```python
from build123d import *

# Parameters (mm, degrees)
SKETCH_2_W           = 80
SKETCH_2_H           = 34
SKETCH_2_R           = 4.05
EXTRUDE_1_DEPTH      = 8
SKETCH_3_R           = 2.55
CUT_EXTRUDE_1_DEPTH  = 88.292611371
CUT_EXTRUDE_2_DEPTH  = 88.292611371
SKETCH_5_R           = 1.55
CUT_EXTRUDE_3_DEPTH  = 88.292611371
CUT_EXTRUDE_5_DEPTH  = 4.5
SKETCH_11_R          = 1.55
CUT_EXTRUDE_7_DEPTH  = 88.292611371
CUT_EXTRUDE_11_DEPTH = 2
CUT_EXTRUDE_13_DEPTH = 6
SKETCH_20_R          = 5.5
CUT_EXTRUDE_14_DEPTH = 88.292611371


with BuildPart() as part:
    # 草图2 → 凸台-拉伸1 (new body)
    with BuildSketch(Plane.XY):
        with Locations((40, 17)):
            Rectangle(SKETCH_2_W, SKETCH_2_H)
        with Locations((7, 8)):
            Circle(SKETCH_2_R, mode=Mode.SUBTRACT)
        with Locations((40, 10)):
            Circle(SKETCH_2_R, mode=Mode.SUBTRACT)
        with Locations((73, 8)):
            Circle(SKETCH_2_R, mode=Mode.SUBTRACT)
    extrude(amount=EXTRUDE_1_DEPTH)

    # 草图3 → 切除-拉伸1 (cut, through all)
    with BuildSketch(Plane.XY.offset(8)):
        with Locations((23, 8)):
            Circle(SKETCH_3_R)
        with Locations((57, 8)):
            Circle(SKETCH_3_R)
    extrude(amount=-CUT_EXTRUDE_1_DEPTH, mode=Mode.SUBTRACT)

    # 草图4 → 切除-拉伸2 (cut, through all)
    with BuildSketch(Plane(origin=(80, 0, 0), x_dir=(0, 0, -1), z_dir=(1, 0, 0))):
        Polygon((-1.5, 32.2), (-2.5, 32.2), (-2.5, 34), (0, 34), (0, 28.8), (-1.5, 28.8), align=None)
    extrude(amount=-CUT_EXTRUDE_2_DEPTH, mode=Mode.SUBTRACT)

    # 草图5 → 切除-拉伸3 (cut, through all)
    with BuildSketch(Plane.XY.offset(8)):
        with Locations((48, 10)):
            Circle(SKETCH_5_R)
        with Locations((32, 10)):
            Circle(SKETCH_5_R)
    extrude(amount=-CUT_EXTRUDE_3_DEPTH, mode=Mode.SUBTRACT)

    # 草图8 → 切除-拉伸5 (cut)
    with BuildSketch(Plane(origin=(0, 0, 0), x_dir=(-1, 0, 0), z_dir=(0, 0, -1))):
        Polygon((-45.15, 8.354551733), (-45.15, 11.645448267), (-48, 13.290896534), (-50.85, 11.645448267), (-50.85, 8.354551733), (-48, 6.709103466), align=None)
        Polygon((-29.15, 8.354551733), (-29.15, 11.645448267), (-32, 13.290896534), (-34.85, 11.645448267), (-34.85, 8.354551733), (-32, 6.709103466), align=None)
    extrude(amount=-CUT_EXTRUDE_5_DEPTH, mode=Mode.SUBTRACT)

    # 草图11 → 切除-拉伸7 (cut, through all)
    with BuildSketch(Plane(origin=(0, 0, 0), x_dir=(-1, 0, 0), z_dir=(0, 0, -1))):
        with Locations((-60, 25)):
            Circle(SKETCH_11_R)
        with Locations((-20, 25)):
            Circle(SKETCH_11_R)
    extrude(amount=-CUT_EXTRUDE_7_DEPTH, mode=Mode.SUBTRACT)

    # 草图19 → 切除-拉伸11 (cut)
    with BuildSketch(Plane(origin=(0, 0, 2.5), x_dir=(-1, 0, 0), z_dir=(0, 0, -1))):
        with BuildLine():
            Line((-25, 34), (-55.247938178, 34))
            Line((-55.247938178, 34), (-55.247938178, 33.2))
            ThreePointArc((-55.247938178, 33.2), (-54.747938178, 32.7), (-54.247938178, 33.2))
            Line((-54.247938178, 33.2), (-26, 33.2))
            ThreePointArc((-26, 33.2), (-25.5, 32.7), (-25, 33.2))
            Line((-25, 33.2), (-25, 34))
        make_face()
    extrude(amount=-CUT_EXTRUDE_11_DEPTH, mode=Mode.SUBTRACT)

    # 草图7 → 切除-拉伸13 (cut)
    with BuildSketch(Plane(origin=(0, 0, 0), x_dir=(-1, 0, 0), z_dir=(0, 0, -1))):
        Polygon((-52.9, 5.632863896), (-52.9, 10.367136104), (-57, 12.734272207), (-61.1, 10.367136104), (-61.1, 5.632863896), (-57, 3.265727793), align=None)
        Polygon((-18.9, 5.632863896), (-18.9, 10.367136104), (-23, 12.734272207), (-27.1, 10.367136104), (-27.1, 5.632863896), (-23, 3.265727793), align=None)
    extrude(amount=-CUT_EXTRUDE_13_DEPTH, mode=Mode.SUBTRACT)

    # 草图20 → 切除-拉伸14 (cut, through all)
    with BuildSketch(Plane(origin=(0, 0, 0), x_dir=(-1, 0, 0), z_dir=(0, 0, -1))):
        with Locations((-40, 10)):
            Circle(SKETCH_20_R)
    extrude(amount=-CUT_EXTRUDE_14_DEPTH, mode=Mode.SUBTRACT)


solid = part.part
```
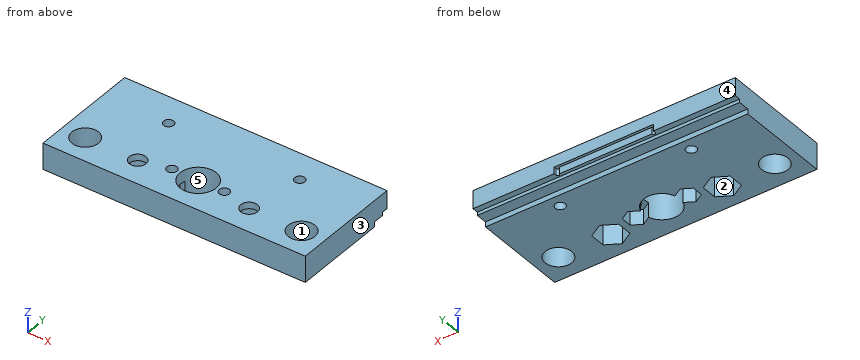
Build history of the part. All positions in model axes, mm. Face numbers are marked on the shaded views. A direction names the side the tool comes from. Round coordinates to 2 decimals unless told otherwise and drop trailing zeros. Write each loop counter-clockwise with the first axis right and the second up, starting at its lowest first coordinate (ties: lowest second). Pieces come first, ordered by that corner, then holes.
1) Mould opens along Y. For the marked faces 3, 4 and 5 say: +Y half, -Y half, draft (parallel to the pull), parting line (faces both ways), or undercut.
2) Band-saw the part on A-A, the plane y = 25. List the corners of the cut face in (x, z).
3) Band-saw the part on C-C, the plane z = 7.25. Give the number of separate pieces and of enclosed holes in the cut face, and give its area (3 significant figures).
4) Band-saw the part on B-B, the plane x = 7. List the corners of the cut face in (y, z), and give its area (3 significant figures).
5) Pin check, flat tips, straight feed: pin 1 (2 mm diameter, centred on x = 46, z = 3, fed in from +Y); pin 2 (3 mm diameter, centred on x = 41.5, y = 20.5, fed in from -Z); pin 3 (4.5 mm diameter, centred on x = 48.5, y = 10, fed in from -Z); pin 4 (0.5 mm diameter, centred on x = 51, y = 33, fed in from -Z). Stop position of each tip, or through.
6) Band-saw the part on D-D, the plane x = 62.5. List the corners of the cut face in (y, z).
7) 3-axis set-ups, long thin cutter, end or side, ignore diameter. For the marked faces 1 and 2: which of +Z, -Z, +X, -X, +Y, -Y reach the whole face in a straight line?
8) Drill centre lines: probe 1 along Y at (x, z) = (23, 6.45); probe 2 along Y at (x, z) = (32, 5.2); probe 3 along X at (y, z) = (12.5, 4.75). Where is each one in solid material? Low to high.
Ans:
1. face 3: draft
1. face 4: +Y half
1. face 5: undercut
2. outline: (0, 0) - (18.45, 0) - (18.45, 8) - (0, 8) - close; (21.55, 0) - (58.45, 0) - (58.45, 8) - (21.55, 8) - close; (61.55, 0) - (80, 0) - (80, 8) - (61.55, 8) - close
3. separate pieces: 1
3. enclosed holes: 9
3. area: 2,450 mm2
4. outline: (0, 0) - (3.95, 0) - (3.95, 8) - (0, 8) - close; (12.05, 0) - (28.8, 0) - (28.8, 1.5) - (32.2, 1.5) - (32.2, 2.5) - (34, 2.5) - (34, 8) - (12.05, 8) - close
4. area: 198 mm2
5. pin 1: stops at y = 33.2
5. pin 2: stops at z = 0
5. pin 3: stops at z = 4.5
5. pin 4: stops at z = 2.5
6. outline: (0, 0) - (28.8, 0) - (28.8, 1.5) - (32.2, 1.5) - (32.2, 2.5) - (34, 2.5) - (34, 8) - (0, 8) - close
7. face 1: +Z, -Z
7. face 2: -Z
8. probe 1: y = 0 to 5.45, 10.55 to 34
8. probe 2: y = 0 to 8.45, 11.55 to 34
8. probe 3: x = 0 to 22.59, 23.41 to 35.1, 44.9 to 56.59, 57.41 to 80
